Verification items for the finished model (mm, model axes). A direction names the side the tool comes from. Coordinates: 2 decimals unless noted, no trailing zeros. Loops run counter-clockwise (first coordinate to the right, second up) from the corner with the lowest first, then second, coordinate; pieces in that order, holes last. Notation, with made-up numbers: (40, 45.25) -> (89, 45.25) arc R17 ccw to (89, 58.25) -> close; hole circle Ø10 at (-0.5, -36). An arc over 180 degrees is marked (long way). Write item = value, one per line.
```python
from build123d import *

# Parameters (mm, degrees)
SKETCH1_W           = 40.64
SKETCH1_H           = 20.32
BOSS_EXTRUDE1_DEPTH = 7.62
SKETCH2_W           = 88.9
SKETCH2_H           = 5.08
BOSS_EXTRUDE2_DEPTH = 12.7
SKETCH3_W           = 88.9
SKETCH3_H           = 5.08
BOSS_EXTRUDE3_DEPTH = 12.7
FILLET1_R           = 7.62
FILLET2_R           = 7.62


with BuildPart() as part:
    # Sketch1 → Boss-Extrude1 (new body)
    with BuildSketch(Plane.XY):
        with BuildLine():
            Line((-44.45, 16.51), (-44.45, 0))
            Line((-44.45, 0), (44.45, 0))
            Line((44.45, 0), (44.45, 16.51))
            ThreePointArc((44.45, 16.51), (35.108257793, 39.328942839), (16.502983922, 55.509674712))
            ThreePointArc((16.502983922, 55.509674712), (0, 59.571022016), (-16.502983922, 55.509674712))
            ThreePointArc((-16.502983922, 55.509674712), (-35.108257793, 39.328942839), (-44.45, 16.51))
        make_face()
        with Locations((0, 38.1)):
            Rectangle(SKETCH1_W, SKETCH1_H, mode=Mode.SUBTRACT)
    extrude(amount=BOSS_EXTRUDE1_DEPTH)

    # Sketch2 → Boss-Extrude2 (add)
    with BuildSketch(Plane(origin=(0, 0, 0), x_dir=(-1, 0, 0), z_dir=(0, 0, -1))):
        with Locations((0, 2.54)):
            Rectangle(SKETCH2_W, SKETCH2_H)
    extrude(amount=BOSS_EXTRUDE2_DEPTH)

    # Sketch3 → Boss-Extrude3 (add)
    with BuildSketch(Plane.XY.offset(7.62)):
        with Locations((0, 2.54)):
            Rectangle(SKETCH3_W, SKETCH3_H)
    extrude(amount=BOSS_EXTRUDE3_DEPTH)

    # Fillet1
    fillet1_edges = [part.edges().sort_by_distance(p)[0] for p in [
        (0, 5.08, 0),
        (-44.45, 2.54, 20.32),
        (44.45, 2.54, 20.32),
    ]]
    fillet(fillet1_edges, radius=FILLET1_R)

    # Fillet2
    fillet2_edges = [part.edges().sort_by_distance(p)[0] for p in [
        (-44.45, 2.54, -12.7),
        (0, 5.08, 7.62),
        (44.45, 2.54, -12.7),
    ]]
    fillet(fillet2_edges, radius=FILLET2_R)


solid = part.part
```
1) Material ranges on line 1 (Z direction, x = 4, y = 15); line 2 (Y direction, x = 33, z = 18.5); line 3 (X direction, y = 33, z = 1.5), recorded low to high.
Ans:
line_1 = 0 to 7.62
line_2 = 0 to 5.08
line_3 = -39.01 to -20.32, 20.32 to 39.01
2) Tool access check on faces 1 (the face through (-44.45, 6, 4)), 2 (the face through (-42.277, 2.797, 18.029)), 3 (the face through (-20.32, 38, 4)), 4 (the face through (-1, 26, 0)), 5 (the face through (-1, 26, 7.62)). Record the directions out of +Z, -Z, +X, -X, +Y, -Y that give a thin tool (end or side, any length) a straight path to the whole face; none if there is none.
Ans:
face_1 = +Z, -Z, -X, +Y, -Y
face_2 = +Z, -X, +Y, -Y
face_3 = +Z, -Z
face_4 = -Z, +X, -X, +Y
face_5 = +Z, +X, -X, +Y
3) Sectioned sample at D-D, the plane x = 23.5. Record the cut outline in (y, z).
Ans:
outline = (0, -12.7) -> (5.08, -12.7) -> (5.08, -7.62) arc R7.62 cw to (12.7, 0) -> (51.12, 0) -> (51.12, 7.62) -> (12.7, 7.62) arc R7.62 cw to (5.08, 15.24) -> (5.08, 20.32) -> (0, 20.32) -> close
4) Release check for a two-part mould opening along X. For faces 6 (the face through (20.32, 38, 4)), 7 (the face through (44.45, 6, 4)), 8 (the face through (0.622, 7.253, 9.911)) record: pulls with the +X half, pulls with the -X half, needs draft (parallel to the pull), parting line crosses it, or undercut.
Ans:
face_6 = undercut
face_7 = pulls with the +X half
face_8 = needs draft
5) Sectioned sample at B-B, the plane y = 47. Record the cut outline in (x, z).
Ans:
outline = (-28.42, 0) -> (-20.32, 0) -> (-20.32, 7.62) -> (-28.42, 7.62) -> close; (20.32, 0) -> (28.42, 0) -> (28.42, 7.62) -> (20.32, 7.62) -> close
6) Sectioned sample at A-A, the plane z = 2. Record the cut outline in (x, y) (3 decimals), plus the area to 3 significant figures.
Ans:
outline = (-44.45, 0) -> (44.45, 0) -> (44.45, 16.51) arc R53.348 ccw to (16.503, 55.51) arc R35.56 ccw to (-16.503, 55.51) arc R53.348 ccw to (-44.45, 16.51) -> close; hole (-20.32, 27.94) -> (20.32, 27.94) -> (20.32, 48.26) -> (-20.32, 48.26) -> close
area = 3,480 mm2
7) Depth check by flat-ended pin: pin 1 Ø5.5 at (x, z) = (-2, 17.5) entering from +Y; pin 2 Ø10 at (y, z) = (46, 4.5) entering from +X; pin 3 Ø12 at (x, z) = (-33.5, -5) entering from +Y. Enter the tip coordinate at first touch or a pass-through.
Ans:
pin_1 = 5.1
pin_2 = 33.86
pin_3 = 45.25
8) Sectioned sample at C-C, the plane x = -12. Record the cut outline in (y, z), plus the area to 3 significant figures.
Ans:
outline = (0, -12.7) -> (5.08, -12.7) -> (5.08, -7.62) arc R7.62 cw to (12.7, 0) -> (27.94, 0) -> (27.94, 7.62) -> (12.7, 7.62) arc R7.62 cw to (5.08, 15.24) -> (5.08, 20.32) -> (0, 20.32) -> close; (48.26, 0) -> (57.49, 0) -> (57.49, 7.62) -> (48.26, 7.62) -> close
area = 437 mm2
